Here's how the part is built. I have some questions about the finished solid (model axes, mm). Face numbers are marked on the shaded views. A direction names the side the tool comes from. Round coordinates to 2 decimals unless told otherwise and drop trailing zeros. Write each loop counter-clockwise with the first axis right and the second up, starting at its lowest first coordinate (ties: lowest second). Pieces come first, ordered by that corner, then holes. Notation, with made-up numbers: (-8, 51) - (21, 51) arc R12 cw to (21, 61) - close; hole circle Ø9 at (33, -26.75). An arc over 180 degrees is marked (long way). Use one line per item in the form item = value. Start each with the question number.
1. I want a section at B-B, the plane y = 26. List the corners of the cut face in (x, z) for me.
2. Will these pins go through, and if not, where does the flat tip stop? pin 1 (1.5 mm diameter, centred on x = 16.5, y = 28, fed in from +Z); pin 2 (18.5 mm diameter, centred on x = 10.5, y = 18.5, fed in from +Z); pin 3 (3 mm diameter, centred on x = 29, z = -1, fed in from -Y).
3. We'd pull the mould along Y, two halves only. Please class the marked faces 1, 2 and 3: +Y half, -Y half, draft (parallel to the pull), parting line (faces both ways), or undercut.
4. If I drill on line 1 along Y through (x, z) = (41, 2.5); line 2 along Y through (x, z) = (3, 2.5); line 3 along X through (y, z) = (27, -0.25), over which ranges is the centre line in solid material (lowest first)?
5. I want a section at C-C, the plane x = 0. List the corners of the cut face in (y, z) for me.
6. I want a section at D-D, the plane y = 0. List the corners of the cut face in (x, z) for me, plus the area to 3 significant figures.
7. Which directions (+Z, -Z, +X, -X, +Y, -Y) give clear straight access to the entire face, cutting with the end or side of a thin tool? Please do the marked faces 4, 5 and 6.
8. I want a section at A-A, the plane z = 0.5. List the corners of the cut face in (x, y) for me, plus the area to 3 significant figures.
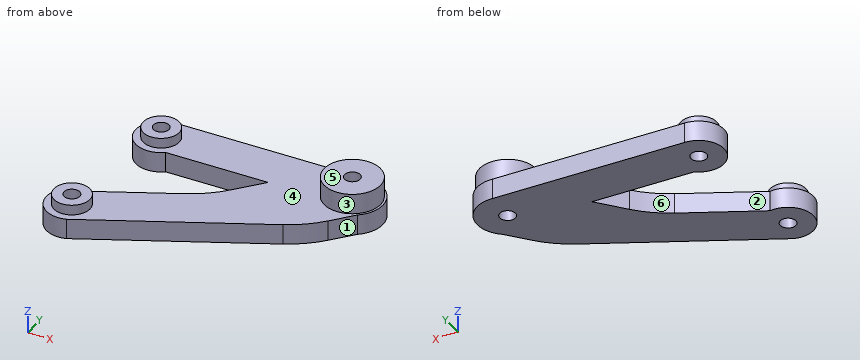
```python
from build123d import *

# Parameters (mm, degrees)
BOSS_EXTRUDE1_DEPTH      = 2
BOSS_EXTRUDE1_DEPTH_BACK = 2
SKETCH2_R                = 1.55
FILLET1_R                = 20
SKETCH7_R                = 5.55
SKETCH7_R_2              = 1.55
BOSS_EXTRUDE4_DEPTH      = 4
SKETCH8_R                = 3.55
SKETCH8_R_2              = 1.55
BOSS_EXTRUDE5_DEPTH      = 2


with BuildPart() as part:
    # Sketch2 → Boss-Extrude1 (new, two sides: drawn at the far end of the back side and taken through both)
    with BuildSketch(Plane.XY.offset(-BOSS_EXTRUDE1_DEPTH_BACK)):
        with BuildLine():
            Line((1.575752274, -4.745208612), (38.598254294, 14.069940073))
            Line((38.598254294, 14.069940073), (44.683748534, 21.26396825))
            ThreePointArc((44.683748534, 21.26396825), (46.605489471, 28.139740122), (40.590896347, 31.986036602))
            Line((40.590896347, 31.986036602), (3, 31))
            ThreePointArc((3, 31), (-1.722747684, 24.35815521), (6.101607472, 22.078261726))
            Line((6.101607472, 22.078261726), (26.170960727, 22.604695486))
            Line((26.170960727, 22.604695486), (19.115779569, 14.264342174))
            Line((19.115779569, 14.264342174), (0.76923556, 4.940473323))
            ThreePointArc((0.76923556, 4.940473323), (-4.982755324, -0.41490888), (1.575752274, -4.745208612))
        make_face()
        Circle(SKETCH2_R, mode=Mode.SUBTRACT)
        with Locations((41, 26)):
            Circle(SKETCH2_R, mode=Mode.SUBTRACT)
        with Locations((3, 26)):
            Circle(SKETCH2_R, mode=Mode.SUBTRACT)
    extrude(amount=BOSS_EXTRUDE1_DEPTH + BOSS_EXTRUDE1_DEPTH_BACK)

    # Fillet1
    fillet1_edges = [part.edges().sort_by_distance(p)[0] for p in [
        (38.598254294, 14.069940073, 0),
        (19.115779569, 14.264342174, 0),
    ]]
    fillet(fillet1_edges, radius=FILLET1_R)

    # Sketch7 → Boss-Extrude4 (add)
    with BuildSketch(Plane(origin=(0, 0, 2), x_dir=(-1, 0, 0), z_dir=(0, 0, -1))):
        with Locations((-41, 26)):
            Circle(SKETCH7_R)
        with Locations(Location((-41, 26, 0), (0, 0, 180))):
            Circle(SKETCH7_R_2, mode=Mode.SUBTRACT)
    extrude(amount=-BOSS_EXTRUDE4_DEPTH)

    # Sketch8 → Boss-Extrude5 (add)
    # profile 1 of 2: a face of its own
    with BuildSketch(Plane.XY.offset(2)):
        with Locations((3, 26)):
            Circle(SKETCH8_R)
        with Locations((3, 26)):
            Circle(SKETCH8_R_2, mode=Mode.SUBTRACT)
    # profile 2 of 2: a face of its own
    with BuildSketch(Plane.XY.offset(2)):
        Circle(SKETCH8_R)
        Circle(SKETCH8_R_2, mode=Mode.SUBTRACT)
    extrude(amount=BOSS_EXTRUDE5_DEPTH)


solid = part.part
```
Model answer:
q1.outline = (-2, -2) - (1.45, -2) - (1.45, 4) - (-0.55, 4) - (-0.55, 2) - (-2, 2) - close; (4.55, -2) - (39.45, -2) - (39.45, 6) - (35.45, 6) - (35.45, 2) - (6.55, 2) - (6.55, 4) - (4.55, 4) - close; (42.55, -2) - (47, -2) - (47, 2) - (46.55, 2) - (46.55, 6) - (42.55, 6) - close
q2.pin_1 = 2
q2.pin_2 = 4
q2.pin_3 = 8.43
q3.face_1 = -Y half
q3.face_2 = undercut
q3.face_3 = parting line
q4.line_1 = 20.45 to 24.45, 27.55 to 31.55
q4.line_2 = -1.9 to 1.9, 22.45 to 24.45, 27.55 to 29.55
q4.line_3 = -1.9 to 1.82, 4.18 to 39.82, 42.18 to 46.92
q5.outline = (-5, -2) - (-1.55, -2) - (-1.55, 4) - (-3.55, 4) - (-3.55, 2) - (-5, 2) - close; (1.55, -2) - (5, -2) - (5, 2) - (3.55, 2) - (3.55, 4) - (1.55, 4) - close; (22, -2) - (30, -2) - (30, 2) - (27.9, 2) - (27.9, 4) - (24.1, 4) - (24.1, 2) - (22, 2) - close
q6.outline = (-5, -2) - (-1.55, -2) - (-1.55, 4) - (-3.55, 4) - (-3.55, 2) - (-5, 2) - close; (1.55, -2) - (10.91, -2) - (10.91, 2) - (3.55, 2) - (3.55, 4) - (1.55, 4) - close
q6.area = 59.3 mm2
q7.face_4 = +Z
q7.face_5 = +Z, +X, -X, +Y, -Y
q7.face_6 = +Z, -Z, -X
q8.outline = (0.77, 4.94) arc R5 ccw (long way) to (1.58, -4.75) - (35, 12.24) arc R20 ccw to (41.21, 17.15) - (44.68, 21.26) arc R6 ccw to (40.59, 31.99) - (3, 31) arc R5 ccw (long way) to (6.1, 22.08) - (26.17, 22.6) - (21.72, 17.35) arc R20 cw to (15.52, 12.43) - close; hole circle Ø3.1 at (0, 0); hole circle Ø3.1 at (3, 26); hole circle Ø3.1 at (41, 26)
q8.area = 908 mm2
